The listing builds one solid part. Answer for the finished solid, in the listing's coordinates (mm). A direction names the side the tool comes from. Round coordinates to 2 decimals unless told otherwise and drop trailing zeros. Order: outer loops, then holes, each group sorted by start corner. A loop starts at its lowest first (then second) coordinate and runs counter-clockwise, first axis right, second up. Notation, with made-up numbers: (-31, 59) - (7, 59) arc R14 cw to (7, 68) - close; hole circle Ø1 at (54.5, 37). An arc over 180 degrees is marked (long way). Use CSV: the item, a comma, the result in double quotes. Start each with the question number.
Item 1: Find section A-A, the plane x = 6.5. Give the vertices of the cut face in (y, z), plus the area to 3 significant figures.
Item 2: Find section B-B, the plane y = 8.5. Give the vertices of the cut face in (x, z) (3 decimals), plus the area to 3 significant figures.
Item 3: For faces 1 (the flat face through (62, 32, 0)), 2 (the cylindrical face through (59.682, 27.437, -0.477)), 3 (the flat face through (26, 0, 0)), determine the directions among +Z, -Z, +X, -X, +Y, -Y from which every point of the face is accessible in a straight line to the end or side of a thin tool.
Item 4: Find section C-C, the plane y = 29. Give the vertices of the cut face in (x, z).
Item 5: Determine the mould class of faces 4 (the cylindrical face through (8.53, 4.93, -11.45)), 5 (the flat face through (0, 5, 0)), 6 (the flat face through (45, 33.5, -1)) for opening direction X: +X half, -X half, draft (parallel to the pull), parting line (faces both ways), or undercut.
Item 6: Flat-ended cylindrical pins translate along their axes: P1, Ø2, axis at x = 52, z = -5, coming from the +Y side; P2, Ø5, axis at x = 62.5, z = -0.5, coming from the +Y side; P3, Ø10, axis at x = 16.5, y = 17.5, coming from the -Z side; P4, Ø1.5, axis at x = 8, z = -0.5, coming from the +Y side. Find the tip coordinate at first contact, or state that the pin passes through.
Item 7: Find section D-D, the plane x = 63. Give the vertices of the cut face in (y, z), plus the area to 3 significant figures.
Item 8: Straight lines are drawn through the part: line 1 along Z through (x, y) = (6.5, 2.5); line 2 along Z through (x, y) = (7.5, 7); line 3 along Y through (x, z) = (28, -12.5). For each, find the intervals that lie inside material, in ascending order. Write a range as [from, to].
```python
from build123d import *

# Parameters (mm, degrees)
BOSS_EXTRUDE1_DEPTH             = 10
SKETCH2_R                       = 12.5
BOSS_EXTRUDE2_DEPTH             = 13
F_10_CLEARANCE_HOLE1_D          = 5.1054
F_10_CLEARANCE_HOLE1_DEPTH      = 135.89
F_10_CLEARANCE_HOLE1_TIP        = 1.533816902
SKETCH6_R                       = 2.2
BOSS_EXTRUDE3_DEPTH             = 9
SKETCH7_R                       = 2.2
BOSS_EXTRUDE4_DEPTH             = 1.5
F_2_56_TAPPED_HOLE1_D           = 1.778
F_2_56_TAPPED_HOLE1_DEPTH       = 6.64
F_2_56_TAPPED_HOLE1_CSINK_D     = 3.048
F_2_56_TAPPED_HOLE1_CSINK_ANGLE = 90
F_2_56_TAPPED_HOLE1_TIP         = 0.53416509


with BuildPart() as part:
    # Sketch1 → Boss-Extrude1 (new body)
    with BuildSketch(Plane(origin=(0, 0, 0), x_dir=(1, 0, 0), z_dir=(0, 1, 0))):
        with BuildLine():
            Line((0, 0), (0, 20))
            Line((0, 20), (13, 20))
            Line((13, 20), (56.387051948, 12.308072526))
            ThreePointArc((56.387051948, 12.308072526), (63.784291449, 8.030390733), (66.705, 0))
            Line((66.705, 0), (0, 0))
        make_face()
    extrude(amount=BOSS_EXTRUDE1_DEPTH)

    # Mirror1: part across plane


with BuildPart() as part_1:
    add(part.part)
    add(part.part.mirror(Plane(origin=(66.705, 10, 0), x_dir=(1, 0, 0), z_dir=(0, 0, -1))))

    # Sketch2 → Boss-Extrude2 (add)
    with BuildSketch(Plane(origin=(0, 10, 0), x_dir=(1, 0, 0), z_dir=(0, 1, 0))):
        with Locations(Location((54.205, 0, 0), (0, 0, 79.946704324))):  # turned: the seam where the file's is
            Circle(SKETCH2_R)
    extrude(amount=BOSS_EXTRUDE2_DEPTH)

    # #10 Clearance Hole1
    with Locations(Plane(origin=(0, 10, 0), x_dir=(1, 0, 0), z_dir=(0, 1, 0))):
        with Locations((6.5, 13), (6.5, -13)):
            Hole(F_10_CLEARANCE_HOLE1_D / 2, depth=F_10_CLEARANCE_HOLE1_DEPTH)
            with Locations((0, 0, -(F_10_CLEARANCE_HOLE1_DEPTH + F_10_CLEARANCE_HOLE1_TIP / 2))):  # 118° drill point
                Cone(0, F_10_CLEARANCE_HOLE1_D / 2, F_10_CLEARANCE_HOLE1_TIP, mode=Mode.SUBTRACT)

    # Sketch6 → Boss-Extrude3 (add)
    with BuildSketch(Plane(origin=(0, 23, 0), x_dir=(1, 0, 0), z_dir=(0, 1, 0))):
        with Locations(Location((61.83, 0, 0), (0, 0, 270))):  # turned: the seam where the file's is
            Circle(SKETCH6_R)
        with Locations(Location((46.58, 0, 0), (0, 0, 270))):  # turned: the seam where the file's is
            Circle(SKETCH6_R)
    extrude(amount=BOSS_EXTRUDE3_DEPTH)

    # Sketch7 → Boss-Extrude4 (add)
    with BuildSketch(Plane(origin=(0, 32, 0), x_dir=(1, 0, 0), z_dir=(0, 1, 0))):
        with Locations(Location((46.58, 0, 0), (0, 0, 270))):  # turned: the seam where the file's is
            Circle(SKETCH7_R)
    extrude(amount=BOSS_EXTRUDE4_DEPTH)

    # #2-56 Tapped Hole1
    with Locations(Plane(origin=(0, 33.5, 0), x_dir=(1, 0, 0), z_dir=(0, 1, 0))):
        with Locations((46.58, 0)):
            CounterSinkHole(F_2_56_TAPPED_HOLE1_D / 2, F_2_56_TAPPED_HOLE1_CSINK_D / 2, depth=F_2_56_TAPPED_HOLE1_DEPTH, counter_sink_angle=F_2_56_TAPPED_HOLE1_CSINK_ANGLE)
            with Locations((0, 0, -(F_2_56_TAPPED_HOLE1_DEPTH + F_2_56_TAPPED_HOLE1_TIP / 2))):  # 118° drill point
                Cone(0, F_2_56_TAPPED_HOLE1_D / 2, F_2_56_TAPPED_HOLE1_TIP, mode=Mode.SUBTRACT)


solid = part_1.part
```
Worked out:
1,outline,"(0, -20) - (10, -20) - (10, -15.55) - (0, -15.55) - close; (0, -10.45) - (10, -10.45) - (10, 10.45) - (0, 10.45) - close; (0, 15.55) - (10, 15.55) - (10, 20) - (0, 20) - close"
1,area,"298 mm²"
2,outline,"(0, -20) - (13, -20) - (56.387, -12.308) arc R12.5 ccw to (56.387, 12.308) - (13, 20) - (0, 20) - close; hole circle Ø5.105 at (6.5, -13); hole circle Ø5.105 at (6.5, 13)"
2,area,"2,070 mm²"
3,face 1,"+Z, -Z, +X, +Y"
3,face 2,"+Y"
3,face 3,"+Z, -Z, +X, -X, -Y"
4,outline,"circle Ø4.4 at (46.58, 0); circle Ø4.4 at (61.83, 0); hole circle Ø1.78 at (46.58, 0)"
5,face 4,"undercut"
5,face 5,"-X half"
5,face 6,"draft"
6,P1,"stops at y = 23"
6,P2,"stops at y = 32"
6,P3,"passes through"
6,P4,"stops at y = 10"
7,outline,"(0, -8.88) - (23, -8.88) - (23, -1.86) - (32, -1.86) - (32, 1.86) - (23, 1.86) - (23, 8.88) - (0, 8.88) - close"
7,area,"442 mm²"
8,line 1,"z = [-20, -15.55], [-10.45, 10.45], [15.55, 20]"
8,line 2,"z = [-20, -15.35], [-10.65, 10.65], [15.35, 20]"
8,line 3,"y = [0, 10]"
